```python
from build123d import *

# Parameters (mm, degrees)
SKETCH_1_W             = 30
SKETCH_1_H             = 6
EXTRUDE_1_DEPTH        = 5
SKETCH_2_R             = 2.25
CUT_EXTRUDE_1_DEPTH    = 6
SKETCH_3_W             = 40
SKETCH_3_H             = 30
EXTRUDE_2_DEPTH        = 5
SKETCH_4_W             = 3
SKETCH_4_H             = 20
CUT_EXTRUDE_2_DEPTH    = 10
SKETCH_7_W             = 10
SKETCH_7_H             = 5
CUT_EXTRUDE_3_DEPTH    = 31
SKETCH_9_W             = 5
SKETCH_9_H             = 5
EXTRUDE_5_DEPTH        = 18
SKETCH_10_W            = 10
SKETCH_10_H            = 20
CUT_EXTRUDE_4_DEPTH    = 18
SKETCH_11_W            = 17
SKETCH_11_H            = 5
EXTRUDE_6_DEPTH        = 0.7
SKETCH_12_W            = 5
SKETCH_12_H            = 5
EXTRUDE_7_DEPTH        = 0.7
SKETCH_13_W            = 26
SKETCH_13_H            = 18
EXTRUDE_8_DEPTH        = 5
HOLE_WIZARD_M3_1_D     = 2.5
HOLE_WIZARD_M3_1_DEPTH = 7.5
HOLE_WIZARD_M3_1_TIP   = 0.751075774
SKETCH_16_W            = 14.26711197
SKETCH_16_H            = 39.299316136
CUT_EXTRUDE_5_DEPTH    = 31
SKETCH_17_W            = 5
SKETCH_17_H            = 26
EXTRUDE_9_DEPTH        = 30.7
SKETCH_18_W            = 5
SKETCH_18_H            = 26
EXTRUDE_10_DEPTH       = 1
SKETCH_20_W            = 26
SKETCH_20_H            = 8
EXTRUDE_11_DEPTH       = 2
HOLE_WIZARD_M4_1_D     = 3.3
HOLE_WIZARD_M4_1_DEPTH = 6
HOLE_WIZARD_M4_1_TIP   = 0.991420021
SKETCH_23_W            = 26
SKETCH_23_H            = 12
CUT_EXTRUDE_6_DEPTH    = 1
HOLE_WIZARD_M3_2_D     = 2.5
HOLE_WIZARD_M3_2_DEPTH = 7.5
HOLE_WIZARD_M3_2_TIP   = 0.751075774


with BuildPart() as part:
    # 草图1 → 凸台-拉伸1 (new body)
    with BuildSketch(Plane.XY):
        with Locations((15, 3)):
            Rectangle(SKETCH_1_W, SKETCH_1_H)
    extrude(amount=EXTRUDE_1_DEPTH)

    # 草图2 → 切除-拉伸1 (cut, through all)
    with BuildSketch(Plane.XY.offset(5)):
        with Locations((22.5, 3)):
            Circle(SKETCH_2_R)
        with Locations((7.5, 3)):
            Circle(SKETCH_2_R)
    extrude(amount=-CUT_EXTRUDE_1_DEPTH, mode=Mode.SUBTRACT)

    # 草图3 → 凸台-拉伸2 (add)
    with BuildSketch(Plane.XY.offset(5)):
        with Locations((10, 21)):
            Rectangle(SKETCH_3_W, SKETCH_3_H)
    extrude(amount=-EXTRUDE_2_DEPTH)

    # 草图4 → 切除-拉伸2 (cut)
    with BuildSketch(Plane.XY.offset(5)):
        with Locations((28.5, 26)):
            Rectangle(SKETCH_4_W, SKETCH_4_H)
    extrude(amount=-CUT_EXTRUDE_2_DEPTH, mode=Mode.SUBTRACT)

    # 草图7 → 切除-拉伸3 (cut, through all)
    with BuildSketch(Plane.XZ.offset(-6)):
        with Locations((-5, 2.5)):
            Rectangle(SKETCH_7_W, SKETCH_7_H)
    extrude(amount=-CUT_EXTRUDE_3_DEPTH, mode=Mode.SUBTRACT)

    # 草图9 → 凸台-拉伸5 (add)
    with BuildSketch(Plane(origin=(0, 36, 0), x_dir=(1, 0, 0), z_dir=(0, 1, 0))):
        with Locations((19.9, -2.5)):
            Rectangle(SKETCH_9_W, SKETCH_9_H)
    extrude(amount=EXTRUDE_5_DEPTH)

    # 草图10 → 切除-拉伸4 (cut)
    with BuildSketch(Plane.XY.offset(5)):
        with Locations((5, 26)):
            Rectangle(SKETCH_10_W, SKETCH_10_H)
    extrude(amount=-CUT_EXTRUDE_4_DEPTH, mode=Mode.SUBTRACT)

    # 草图11 → 凸台-拉伸6 (add)
    with BuildSketch(Plane(origin=(0, 36, 0), x_dir=(1, 0, 0), z_dir=(0, 1, 0))):
        with Locations((18.5, -2.5)):
            Rectangle(SKETCH_11_W, SKETCH_11_H)
    extrude(amount=EXTRUDE_6_DEPTH)

    # 草图12 → 凸台-拉伸7 (add)
    with BuildSketch(Plane(origin=(0, 54, 0), x_dir=(1, 0, 0), z_dir=(0, 1, 0))):
        with Locations((19.9, -2.5)):
            Rectangle(SKETCH_12_W, SKETCH_12_H)
    extrude(amount=EXTRUDE_7_DEPTH)

    # 草图13 → 凸台-拉伸8 (add)
    with BuildSketch(Plane.ZY.offset(-17.4)):
        with Locations((2.5, 45.7)):
            Rectangle(SKETCH_13_W, SKETCH_13_H)
    extrude(amount=-EXTRUDE_8_DEPTH)

    # M3 螺纹孔1
    with Locations(Plane(origin=(22.4, 0, 0), x_dir=(0, 0, -1), z_dir=(1, 0, 0))):
        with Locations((-10, 40.2), (5, 40.2), (5, 51.2), (-10, 51.2)):
            Hole(HOLE_WIZARD_M3_1_D / 2, depth=HOLE_WIZARD_M3_1_DEPTH)
            with Locations((0, 0, -(HOLE_WIZARD_M3_1_DEPTH + HOLE_WIZARD_M3_1_TIP / 2))):  # 118° drill point
                Cone(0, HOLE_WIZARD_M3_1_D / 2, HOLE_WIZARD_M3_1_TIP, mode=Mode.SUBTRACT)

    # 草图16 → 切除-拉伸5 (cut, through all)
    with BuildSketch(Plane(origin=(30, 0, 0), x_dir=(0, 0, -1), z_dir=(1, 0, 0))):
        with Locations((-7.133555985, 17.050341932)):
            Rectangle(SKETCH_16_W, SKETCH_16_H)
    extrude(amount=-CUT_EXTRUDE_5_DEPTH, mode=Mode.SUBTRACT)

    # 草图17 → 凸台-拉伸9 (add)
    with BuildSketch(Plane.XZ.offset(-36.7)):
        with Locations((19.9, 2.5)):
            Rectangle(SKETCH_17_W, SKETCH_17_H)
    extrude(amount=EXTRUDE_9_DEPTH)

    # 草图18 → 凸台-拉伸10 (add)
    with BuildSketch(Plane.XZ.offset(-6)):
        with Locations((19.9, 2.5)):
            Rectangle(SKETCH_18_W, SKETCH_18_H)
    extrude(amount=EXTRUDE_10_DEPTH)

    # 草图20 → 凸台-拉伸11 (add)
    with BuildSketch(Plane.ZY.offset(-17.4)):
        with Locations((2.5, 9)):
            Rectangle(SKETCH_20_W, SKETCH_20_H)
    extrude(amount=EXTRUDE_11_DEPTH)

    # M4 螺纹孔1
    with Locations(Plane(origin=(0, 5, 0), x_dir=(-1, 0, 0), z_dir=(0, -1, 0))):
        with Locations((-18.9, -7.640506964), (-18.9, 3.359493036)):
            Hole(HOLE_WIZARD_M4_1_D / 2, depth=HOLE_WIZARD_M4_1_DEPTH)
            with Locations((0, 0, -(HOLE_WIZARD_M4_1_DEPTH + HOLE_WIZARD_M4_1_TIP / 2))):  # 118° drill point
                Cone(0, HOLE_WIZARD_M4_1_D / 2, HOLE_WIZARD_M4_1_TIP, mode=Mode.SUBTRACT)

    # 草图23 → 切除-拉伸6 (cut)
    with BuildSketch(Plane(origin=(22.4, 0, 0), x_dir=(0, 0, -1), z_dir=(1, 0, 0))):
        with Locations((-2.5, 24.7)):
            Rectangle(SKETCH_23_W, SKETCH_23_H)
    extrude(amount=-CUT_EXTRUDE_6_DEPTH, mode=Mode.SUBTRACT)

    # M3 螺纹孔2
    with Locations(Plane(origin=(21.4, 0, 0), x_dir=(0, 0, -1), z_dir=(1, 0, 0))):
        with Locations((2.955672884, 23.7)):
            Hole(HOLE_WIZARD_M3_2_D / 2, depth=HOLE_WIZARD_M3_2_DEPTH)
            with Locations((0, 0, -(HOLE_WIZARD_M3_2_DEPTH + HOLE_WIZARD_M3_2_TIP / 2))):  # 118° drill point
                Cone(0, HOLE_WIZARD_M3_2_D / 2, HOLE_WIZARD_M3_2_TIP, mode=Mode.SUBTRACT)


solid = part.part
```
The model under review builds one solid part; all positions refer to its coordinate system, in mm. A direction names the side the tool comes from. Round coordinates to 2 decimals unless told otherwise and drop trailing zeros. Write each loop counter-clockwise with the first axis right and the second up, starting at its lowest first coordinate (ties: lowest second). Pieces come first, ordered by that corner, then holes. Notation, with made-up numbers: (7.25, -27) - (30.25, -27) arc R24 cw to (30.25, 6) - close; hole circle Ø1 at (36.25, 21.25). An arc over 180 degrees is marked (long way). Answer as CSV lines item,"result". Start each with the question number.
(1) Draft analysis for pull direction X (two halves, no side actions). For faces 1 (the flat face through (19, 5, 2)), 2 (the flat face through (17.4, 34, 2)), 3 (the cylindrical face through (20.474, 8.042, -3.855)), state which applies: pulls with the +X half, pulls with the -X half, needs draft (parallel to the pull), parting line crosses it, or undercut.
(2) We need section B-B on y = 23.7. State the section outline as (x, z) points, plus the area to 3 significant figures.
(3) To check wall thickness, follow line 1 (Y direction, x = 18.4, z = 10); line 2 (Z direction, x = 18.9, y = 7.7); line 3 (Y direction, x = 21.75, z = 3.75). State the ranges of each line that lie inside material, in increasing order.
(4) We need section A-A on y = 40.2. State the section outline as (x, z) points.
(5) We need section C-C on z = -8.5. State the section outline as (x, y) points, plus the area to 4 significant figures.
(6) For faces 4 (the cylindrical face through (20.474, 8.042, 7.145)), 5 (the flat face through (22, 18.7, 3)), 6 (the flat face through (16, 13, 2)), list the 3-axis set-ups (+Z, -Z, +X, -X, +Y, -Y) from which the entire face can be reached by the end or side of a thin tool; tool diameter is ignored.
(7) We need section D-D on x = 20. Give the number of separate pieces and of enclosed holes in the cut face, plus the area to 3 significant figures.
(8) For pin 1 Ø1 at (x, z) = (17, 3) entering from +Y; pin 2 Ø1 at (y, z) = (26, 10) entering from -X; pin 3 Ø2 at (y, z) = (51.2, 10) entering from -X; pin 4 Ø3.5 at (y, z) = (23, 7) entering from +X, all flat-tipped, find the tip position at first contact; note any pin that passes through.
Worked answers:
1,face 1,"needs draft"
1,face 2,"pulls with the -X half"
1,face 3,"undercut"
2,outline,"(17.4, -10.5) - (21.4, -10.5) - (21.4, -4.21) - (17.4, -4.21) - close; (17.4, -1.71) - (21.4, -1.71) - (21.4, 15.5) - (17.4, 15.5) - close"
2,area,"94.0 mm²"
3,line 1,"5 to 38.95, 41.45 to 49.95, 52.45 to 54.7"
3,line 2,"-10.5 to -5.01, -1.71 to 5.99, 9.29 to 15.5"
3,line 3,"5 to 18.7, 30.7 to 54.7"
4,outline,"(17.4, -10.5) - (22.4, -10.5) - (22.4, -6.25) - (17.4, -6.25) - close; (17.4, -3.75) - (22.4, -3.75) - (22.4, 8.75) - (17.4, 8.75) - close; (17.4, 11.25) - (22.4, 11.25) - (22.4, 15.5) - (17.4, 15.5) - close"
5,outline,"(15.4, 5) - (22.4, 5) - (22.4, 18.7) - (21.4, 18.7) - (21.4, 30.7) - (22.4, 30.7) - (22.4, 54.7) - (17.4, 54.7) - (17.4, 13) - (15.4, 13) - close"
5,area,"252.5 mm²"
6,face 4,"-Y"
6,face 5,"+Z, -Z, +X"
6,face 6,"+Z, -Z, -X, +Y"
7,separate pieces,"1"
7,enclosed holes,"5"
7,area,"1,240 mm²"
8,pin 1,"y = 54.7"
8,pin 2,"x = 17.4"
8,pin 3,"through"
8,pin 4,"x = 21.4"
